```python
from build123d import *

# Parameters (mm, degrees)
F1_DEPTH = 38.1
F3_DEPTH = 27.94
F4_R     = 5.08


with BuildPart() as f1:
    # F0 (on Front) → F1 (new body, symmetric)
    with BuildSketch(Plane.XZ):
        Polygon((0, 25.4), (0, 0), (60.125147, 0), (60.125147, 9.248371), (50.8, 25.4), align=None)
    extrude(amount=F1_DEPTH, both=True)

    # F2 (on Front) → F3 (cut, symmetric)
    with BuildSketch(Plane.XZ):
        Polygon((43.762105, 25.4), (7.93214, 25.4), (12.838667, 9.5122), (43.762105, 9.5122), align=None)
    extrude(amount=F3_DEPTH, both=True, mode=Mode.SUBTRACT)

    # F4
    f4_edges = [f1.edges().sort_by_distance(p)[0] for p in [
        (0, -38.1, 12.7),
        (60.125147, -38.1, 4.624185),
        (60.125147, 38.1, 4.624185),
        (0, 38.1, 12.7),
    ]]
    fillet(f4_edges, radius=F4_R)


solid = f1.part
```
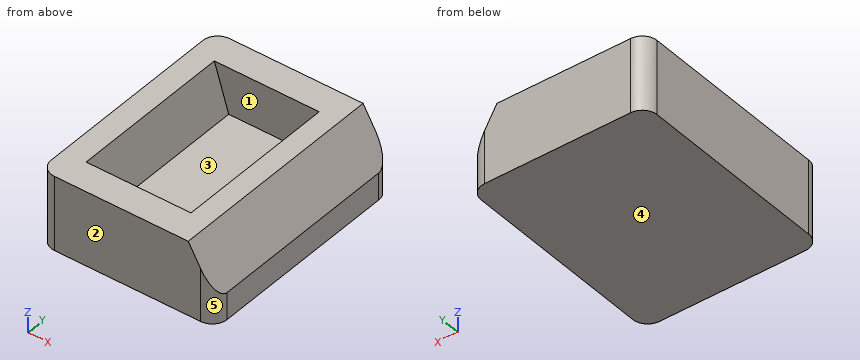
Geometry check sheet. Reference: the model listing, model coordinates, mm. Face numbers are marked on the shaded views. A direction names the side the tool comes from. Give positions to 0.01 mm unless a question says otherwise; leave off trailing zeros. Order: outer loops, then holes, each group sorted by start corner. A loop starts at its lowest first (then second) coordinate and runs counter-clockwise, first axis right, second up.
1. Section check D-D, the plane x = 11.5. Enter the section's corners in (y, z).
2. Access from +Z, -Z, +X, -X, +Y, -Y to the whole of each face (thin tool, end or side, straight path). Record for the marked faces 1 and 2.
3. Section check B-B, the plane y = -29. Enter the section's corners in (x, z).
4. Gauge pin test, flat end, axial feed: pin 1 Ø2 at (x, y) = (24, -19.5) entering from +Z. Record the tip position at first contact, or that the pin passes through.
5. Release check for a two-part mould opening along X. For the marked faces 3, 4 and 5 record: pulls with the +X half, pulls with the -X half, needs draft (parallel to the pull), parting line crosses it, or undercut.
6. Section check A-A, the plane z = 19.75. Enter the section's corners in (x, y), and give its area (3 significant figures).
7. Section check C-C, the plane x = 31.5. Enter the section's corners in (y, z), and give its area (3 significant figures).
8. Thickness scan on L1, parallel to Y at x = 14, z = 24; L2, parallel to Z at x = 16, y = -12; L3, parallel to X at y = -2, z = 20.5. Record the ranges inside material, lowest first.
Values follow:
1. outline: (-38.1, 0) - (38.1, 0) - (38.1, 25.4) - (27.94, 25.4) - (27.94, 13.85) - (-27.94, 13.85) - (-27.94, 25.4) - (-38.1, 25.4) - close
2. face 1: +Z
2. face 2: +Z, -Z, +X, -X, -Y
3. outline: (0, 0) - (60.13, 0) - (60.13, 9.25) - (50.8, 25.4) - (0, 25.4) - close
4. pin 1: stops at z = 9.51
5. face 3: undercut
5. face 4: needs draft
5. face 5: pulls with the +X half
6. outline: (0, -33.02) arc R5.08 ccw to (5.08, -38.1) - (54.06, -38.1) - (54.06, 38.1) - (5.08, 38.1) arc R5.08 ccw to (0, 33.02) - close; hole (9.68, -27.94) - (43.76, -27.94) - (43.76, 27.94) - (9.68, 27.94) - close
6. area: 2,200 mm2
7. outline: (-38.1, 0) - (38.1, 0) - (38.1, 25.4) - (27.94, 25.4) - (27.94, 9.51) - (-27.94, 9.51) - (-27.94, 25.4) - (-38.1, 25.4) - close
7. area: 1,050 mm2
8. L1: y = -38.1 to -27.94, 27.94 to 38.1
8. L2: z = 0 to 9.51
8. L3: x = 0 to 9.45, 43.76 to 53.63
